Here's how the part is built. I have some questions about the finished solid (model axes, mm). A direction names the side the tool comes from. Round coordinates to 2 decimals unless told otherwise and drop trailing zeros. Order: outer loops, then holes, each group sorted by start corner. A loop starts at its lowest first (then second) coordinate and runs counter-clockwise, first axis right, second up. Notation, with made-up numbers: (59.25, -23) -> (99.25, -23) arc R28 cw to (99.25, -4) -> close; hole circle Ø5 at (-40, -10). An arc over 180 degrees is marked (long way). Answer in a Markdown table with one row per item.
```python
from build123d import *

# Parameters (mm, degrees)
BOSS_EXTRUDE1_DEPTH             = 8.89
BOSS_EXTRUDE1_DEPTH_BACK        = 8.89
F_1_4_0_25_DIAMETER_SLOT1_D     = 6.35
F_1_4_0_25_DIAMETER_SLOT1_DEPTH = 9.652
F_1_4_0_25_DIAMETER_SLOT1_TIP   = 1.907732465
TAP_DRILL_FOR_4_40_TAP2_D       = 2.2606
FILLET1_R                       = 2.54
F_10_32_TAPPED_HOLE1_D          = 4.0386


with BuildPart() as part:
    # Sketch1 → Boss-Extrude1 (new, two sides: drawn at the far end of the back side and taken through both)
    with BuildSketch(Plane.XY.offset(-BOSS_EXTRUDE1_DEPTH_BACK)):
        with BuildLine():
            Line((12.698670317, 100.803292467), (12.698670317, 89.373292467))
            Line((12.698670317, 89.373292467), (-12.698670317, 89.373292467))
            Line((-12.698670317, 89.373292467), (-12.698670317, 100.803292467))
            ThreePointArc((-12.698670317, 100.803292467), (0, 101.6), (12.698670317, 100.803292467))
        make_face()
    extrude(amount=BOSS_EXTRUDE1_DEPTH + BOSS_EXTRUDE1_DEPTH_BACK)

    # 1/4 (0.25) Diameter Slot1
    with Locations(Plane(origin=(0, 89.373292467, 0), x_dir=(-1, 0, 0), z_dir=(0, -1, 0))):
        with Locations((0, 0)):
            Hole(F_1_4_0_25_DIAMETER_SLOT1_D / 2, depth=F_1_4_0_25_DIAMETER_SLOT1_DEPTH)
            with Locations((0, 0, -(F_1_4_0_25_DIAMETER_SLOT1_DEPTH + F_1_4_0_25_DIAMETER_SLOT1_TIP / 2))):  # 118° drill point
                Cone(0, F_1_4_0_25_DIAMETER_SLOT1_D / 2, F_1_4_0_25_DIAMETER_SLOT1_TIP, mode=Mode.SUBTRACT)

    # Tap Drill for #4-40 Tap2 (through all)
    with Locations(Plane(origin=(0, 89.373292467, 0), x_dir=(-1, 0, 0), z_dir=(0, -1, 0))):
        with Locations((8.888670317, 0), (-8.888670317, 0)):
            Hole(TAP_DRILL_FOR_4_40_TAP2_D / 2)

    # Fillet1
    fillet1_edges = [part.edges().sort_by_distance(p)[0] for p in [
        (12.698670317, 95.088292467, -8.89),
        (-12.698670317, 95.088292467, 8.89),
        (12.698670317, 95.088292467, 8.89),
        (-12.698670317, 95.088292467, -8.89),
    ]]
    fillet(fillet1_edges, radius=FILLET1_R)

    # #10-32 Tapped Hole1 (through all)
    with Locations(Plane(origin=(0, 0, -8.89), x_dir=(-1, 0, 0), z_dir=(0, 0, -1))):
        with Locations((0, 95.723292467)):
            Hole(F_10_32_TAPPED_HOLE1_D / 2)


solid = part.part
```
1. Suppose I cut it at A-A on y = 95. Write out the boundary of the cut face in (x, z) (3 decimals).
Numbers:
| item | result |
|---|---|
| outline | (-12.699, -6.35) arc R2.54 ccw to (-10.159, -8.89) -> (-1.885, -8.89) -> (-1.885, -2.555) arc R3.175 cw to (-1.885, 2.555) -> (-1.885, 8.89) -> (-10.159, 8.89) arc R2.54 ccw to (-12.699, 6.35) -> close; (1.885, -8.89) -> (10.159, -8.89) arc R2.54 ccw to (12.699, -6.35) -> (12.699, 6.35) arc R2.54 ccw to (10.159, 8.89) -> (1.885, 8.89) -> (1.885, 2.555) arc R3.175 cw to (1.885, -2.555) -> close; hole circle Ø2.261 at (-8.889, 0); hole circle Ø2.261 at (8.889, 0) |
2. For faces 4 (the face through (-3.17, 94.27, -0.14)), 5 (the face through (-2, 96, 6)), which set-ups out of +Z, -Z, +X, -X, +Y, -Y let a thin tool reach every point of the face, with its end or its side?
Numbers:
| item | result |
|---|---|
| face 4 | -Y |
| face 5 | +Z, -Z |
3. For pin 1 Ø3.5 at (x, y) = (0, 95.72) entering from +Z; pin 2 Ø10 at (x, z) = (-7.5, 0) entering from +Y; pin 3 Ø3 at (x, z) = (8.89, 0) entering from +Y; pin 4 Ø1.5 at (x, z) = (5, 3.5) entering from +Y, each with a flat end and sliding along its axis, tell me the tip position at first contact or that it passes through.
Numbers:
| item | result |
|---|---|
| pin 1 | passes through |
| pin 2 | stops at y = 101.57 |
| pin 3 | stops at y = 101.33 |
| pin 4 | stops at y = 101.51 |
4. We'd pull the mould along X, two halves only. Please class faces 1 (the face through (0.12, 100.6, 0.54)), 2 (the face through (-0.2, 101.6, -0.1)), 3 (the face through (2.4, 95.6, -8.89)): released by +X, released by -X, zero draft, split by the parting line, or undercut.
Numbers:
| item | result |
|---|---|
| face 1 | undercut |
| face 2 | split by the parting line |
| face 3 | zero draft |
5. Please list where these lines run through material, in increasing order: line 1 along Y through (x, z) = (0, -6.5); line 2 along Z through (x, y) = (-9, 91.75); line 3 along X through (y, z) = (94, -2).
Numbers:
| item | result |
|---|---|
| line 1 | y = 89.37 to 93.7, 97.74 to 101.6 |
| line 2 | z = -8.89 to -1.12, 1.12 to 8.89 |
| line 3 | x = -12.7 to -2.47, 2.47 to 12.7 |
6. Suppose I cut it at B-B on z = -4.75. Write out the boundary of the cut face in (x, y), then the cut area to 3 significant figures.
Numbers:
| item | result |
|---|---|
| outline | (-12.7, 89.37) -> (12.7, 89.37) -> (12.7, 100.8) arc R101.6 ccw to (-12.7, 100.8) -> close; hole circle Ø4.04 at (0, 95.72) |
| area | 291 mm2 |
